Here's how the part is built. I have some questions about the finished solid (model axes, mm). A direction names the side the tool comes from. Coordinates: 2 decimals unless noted, no trailing zeros. Order: outer loops, then holes, each group sorted by start corner. A loop starts at its lowest first (then second) coordinate and runs counter-clockwise, first axis right, second up. Notation, with made-up numbers: (6, 64) - (15, 64) arc R29 ccw to (15, 95) - close; hole circle Ø9 at (-1.5, -16.75). An arc over 180 degrees is marked (long way). Answer as CSV lines item,"result". Start each with the question number.
Item 1: We'd pull the mould along Z, two halves only. Please class faces 6 (the face through (0, 0, 20)), 7 (the face through (-4, 0, 30)), 8 (the face through (-3.06, 0.87, 31.9)): pulls with the +Z half, pulls with the -Z half, needs draft (parallel to the pull), parting line crosses it, or undercut.
Item 2: Imagine slicing it at B-B on y = 2. Count the separate pieces of the cut face and the enclosed holes in it, and give its area (3 significant figures).
Item 3: Imagine slicing it at C-C on z = 29. List the corners of the cut face in (x, y) for me, and give its area (3 significant figures).
Item 4: On a 3-axis mill with a long thin cutter (end or side, diameter ignored), from which of +Z, -Z, +X, -X, +Y, -Y can I reach the whole of each face in a straight line? I mean faces 1 (the face through (3.34, 1.05, 9.86)), 2 (the face through (-3, 4, 30)), 3 (the face through (-3, 0, 40)), 4 (the face through (3.7, 0.1, 20)), 5 (the face through (2.1, 0, 30)). Say none if no direction works.
Item 5: I'm going to push flat-ended pins straight in: pin 1 (1.3 mm diameter, centred on x = 0.5, y = 1, fed in from +Z); pin 2 (1.5 mm diameter, centred on y = -2, z = 10, fed in from +X); pin 3 (3 mm diameter, centred on y = 0.5, z = 5, fed in from +X). Where does each tip first touch, or does it pass through?
Item 6: Imagine slicing it at A-A on x = 0. List the corners of the cut face in (y, z) for me, and give its area (3 significant figures).
Item 7: I need wall thicknesses on line 1 (Z direction, x = 0, y = 2); line 2 (X direction, y = -2.25, z = 27); line 3 (Z direction, x = 0.75, y = 2.75). Which ranges of each line are inside material? Lowest first, please.
Item 8: Imagine slicing it at D-D on z = 23.5. List the corners of the cut face in (x, y) for me, and give its area (3 significant figures).
from build123d import *

# Parameters (mm, degrees)
SKETCH1_R               = 3.5
BOSS_EXTRUDE1_DEPTH     = 20
SKETCH2_R               = 1.6
CUT_EXTRUDE1_DEPTH      = 4.5
CUT_EXTRUDE1_DEPTH_BACK = 4.5
SKETCH3_W               = 8
SKETCH3_H               = 8
BOSS_EXTRUDE2_DEPTH     = 20
SKETCH4_W               = 4.2
SKETCH4_H               = 8
CUT_EXTRUDE2_DEPTH      = 20
SKETCH5_R               = 1.6
CUT_EXTRUDE3_DEPTH      = 9


with BuildPart() as part:
    # Sketch1 → Boss-Extrude1 (new body)
    with BuildSketch(Plane.XY):
        Circle(SKETCH1_R)
    extrude(amount=BOSS_EXTRUDE1_DEPTH)

    # Sketch2 → Cut-Extrude1 (cut, two sides)
    with BuildSketch(Plane(origin=(0, 0, 0), x_dir=(1, 0, 0), z_dir=(0, 1, 0))) as cut_extrude1_sk:
        with Locations((0, -3)):
            Circle(SKETCH2_R)
        with Locations((0, -16)):
            Circle(SKETCH2_R)
    extrude(amount=CUT_EXTRUDE1_DEPTH, mode=Mode.SUBTRACT)
    extrude(cut_extrude1_sk.sketch, amount=-CUT_EXTRUDE1_DEPTH_BACK, mode=Mode.SUBTRACT)

    # Sketch3 → Boss-Extrude2 (add)
    with BuildSketch(Plane.XY.offset(20)):
        Rectangle(SKETCH3_W, SKETCH3_H)
    extrude(amount=BOSS_EXTRUDE2_DEPTH)

    # Sketch4 → Cut-Extrude2 (cut)
    with BuildSketch(Plane.XY.offset(40)):
        Rectangle(SKETCH4_W, SKETCH4_H)
    extrude(amount=-CUT_EXTRUDE2_DEPTH, mode=Mode.SUBTRACT)

    # Sketch5 → Cut-Extrude3 (cut, through all)
    with BuildSketch(Plane.ZY.offset(4)):
        with Locations((33.5, 0.8)):
            Circle(SKETCH5_R)
        with Locations((23.5, 0.8)):
            Circle(SKETCH5_R)
    extrude(amount=-CUT_EXTRUDE3_DEPTH, mode=Mode.SUBTRACT)


solid = part.part
Responses:
1,face 6,"pulls with the +Z half"
1,face 7,"needs draft"
1,face 8,"undercut"
2,separate pieces,"5"
2,enclosed holes,"2"
2,area,"159 mm^2"
3,outline,"(-4, -4) - (-2.1, -4) - (-2.1, 4) - (-4, 4) - close; (2.1, -4) - (4, -4) - (4, 4) - (2.1, 4) - close"
3,area,"30.4 mm^2"
4,face 1,"-Z"
4,face 2,"+Z, -Z, +X, -X, +Y"
4,face 3,"+Z, +X, -X, +Y, -Y"
4,face 4,"-Z, +X"
4,face 5,"+Z, +Y, -Y"
5,pin 1,"stops at z = 20"
5,pin 2,"stops at x = 3.27"
5,pin 3,"stops at x = 3.5"
6,outline,"(-3.5, 0) - (3.5, 0) - (3.5, 1.4) - (-3.5, 1.4) - close; (-3.5, 4.6) - (3.5, 4.6) - (3.5, 14.4) - (-3.5, 14.4) - close; (-3.5, 17.6) - (3.5, 17.6) - (3.5, 20) - (-3.5, 20) - close"
6,area,"95.2 mm^2"
7,line 1,"z = 0 to 1.4, 4.6 to 14.4, 17.6 to 20"
7,line 2,"x = -4 to -2.1, 2.1 to 4"
7,line 3,"z = 0 to 1.59, 4.41 to 14.59, 17.41 to 20"
8,outline,"(-4, -4) - (-2.1, -4) - (-2.1, -0.8) - (-4, -0.8) - close; (-4, 2.4) - (-2.1, 2.4) - (-2.1, 4) - (-4, 4) - close; (2.1, -4) - (4, -4) - (4, -0.8) - (2.1, -0.8) - close; (2.1, 2.4) - (4, 2.4) - (4, 4) - (2.1, 4) - close"
8,area,"18.2 mm^2"
